Geometry: final body of the model. Coordinates: model frame, mm. Round coordinates to 2 decimals unless told otherwise and drop trailing zeros. Write each loop counter-clockwise with the first axis right and the second up, starting at its lowest first coordinate (ties: lowest second). Pieces come first, ordered by that corner, then holes. Notation, with made-up numbers: (65, -32) - (77, -32) arc R25 ccw to (77, 7) - close; hole circle Ø11 at (-23, -18.5). An arc over 180 degrees is marked (long way). Write each question's results on one line, items separated by ' | '.
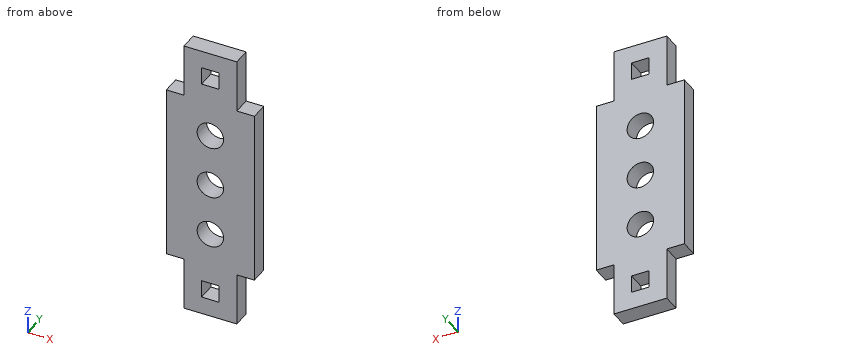
from build123d import *

# Parameters (mm, degrees)
CYLINDER005_R          = 2.25
CYLINDER005_DEPTH      = 3
CYLINDER005_ROLL_ANGLE = 90
CYLINDER006_R          = 2.25
CYLINDER006_DEPTH      = 3
CYLINDER006_ROLL_ANGLE = 90
CYLINDER004_R          = 2.25
CYLINDER004_DEPTH      = 3
CYLINDER004_ROLL_ANGLE = 90
BOX011_W               = 15
BOX011_H               = 3
BOX011_DEPTH           = 30
BOX010_W               = 3
BOX010_H               = 3
BOX010_DEPTH           = 3
BOX009_W               = 9
BOX009_H               = 3
BOX009_DEPTH           = 9
BOX013_W               = 3
BOX013_H               = 3
BOX013_DEPTH           = 3
BOX012_W               = 9
BOX012_H               = 3
BOX012_DEPTH           = 9


with BuildPart() as cylinder005:
    # Cylinder005 → Cylinder005 (new body)
    with BuildSketch(Plane.XY):
        Circle(CYLINDER005_R)
    extrude(amount=CYLINDER005_DEPTH)


with BuildPart() as cylinder005_1:
    # Cylinder005 roll: moved
    add(cylinder005.part.rotate(Axis((0, 0, 0), (1, 0, 0)), CYLINDER005_ROLL_ANGLE))


with BuildPart() as cylinder005_2:
    # Cylinder005 placement: moved
    add(cylinder005_1.part.moved(Location((0, -63, -3))))


with BuildPart() as cylinder006:
    # Cylinder006 → Cylinder006 (new body)
    with BuildSketch(Plane.XY):
        Circle(CYLINDER006_R)
    extrude(amount=CYLINDER006_DEPTH)


with BuildPart() as cylinder006_1:
    # Cylinder006 roll: moved
    add(cylinder006.part.rotate(Axis((0, 0, 0), (1, 0, 0)), CYLINDER006_ROLL_ANGLE))


with BuildPart() as cylinder006_2:
    # Cylinder006 placement: moved
    add(cylinder006_1.part.moved(Location((0, -63, -21))))


with BuildPart() as cylinder004:
    # Cylinder004 → Cylinder004 (new body)
    with BuildSketch(Plane.XY):
        Circle(CYLINDER004_R)
    extrude(amount=CYLINDER004_DEPTH)


with BuildPart() as cylinder004_1:
    # Cylinder004 roll: moved
    add(cylinder004.part.rotate(Axis((0, 0, 0), (1, 0, 0)), CYLINDER004_ROLL_ANGLE))


with BuildPart() as cylinder004_2:
    # Cylinder004 placement: moved
    add(cylinder004_1.part.moved(Location((0, -63, -12))))


with BuildPart() as cube011:
    # Box011 → Box011 (new body)
    with BuildSketch(Plane(origin=(-7.5, -66, -27), x_dir=(1, 0, 0), z_dir=(0, 0, 1))):
        with Locations((7.5, 1.5)):
            Rectangle(BOX011_W, BOX011_H)
    extrude(amount=BOX011_DEPTH)


with BuildPart() as cube010:
    # Box010 → Box010 (new body)
    with BuildSketch(Plane(origin=(-1.5, -66, 6), x_dir=(1, 0, 0), z_dir=(0, 0, 1))):
        with Locations((1.5, 1.5)):
            Rectangle(BOX010_W, BOX010_H)
    extrude(amount=BOX010_DEPTH)


with BuildPart() as cut010:
    # Box009 → Box009 (new body)
    with BuildSketch(Plane(origin=(-4.5, -66, 3), x_dir=(1, 0, 0), z_dir=(0, 0, 1))):
        with Locations((4.5, 1.5)):
            Rectangle(BOX009_W, BOX009_H)
    extrude(amount=BOX009_DEPTH)

    # Cut010: cut Cube010
    add(cube010.part, mode=Mode.SUBTRACT)


with BuildPart() as cube013:
    # Box013 → Box013 (new body)
    with BuildSketch(Plane(origin=(-1.5, -66, 6), x_dir=(1, 0, 0), z_dir=(0, 0, 1))):
        with Locations((1.5, 1.5)):
            Rectangle(BOX013_W, BOX013_H)
    extrude(amount=BOX013_DEPTH)


with BuildPart() as pitchringconnector:
    # Box012 → Box012 (new body)
    with BuildSketch(Plane(origin=(-4.5, -66, 3), x_dir=(1, 0, 0), z_dir=(0, 0, 1))):
        with Locations((4.5, 1.5)):
            Rectangle(BOX012_W, BOX012_H)
    extrude(amount=BOX012_DEPTH)

    # Cut011: cut Cube013
    add(cube013.part, mode=Mode.SUBTRACT)


with BuildPart() as pitchringconnector_1:
    # Cut011 placement: moved
    add(pitchringconnector.part.moved(Location((0, 0, -39))))

    # Fusion: union Cube011, Cut010
    add(cube011.part)
    add(cut010.part)

    # Cut012: cut Cylinder004
    add(cylinder004_2.part, mode=Mode.SUBTRACT)

    # Cut013: cut Cylinder006
    add(cylinder006_2.part, mode=Mode.SUBTRACT)

    # Cut014: cut Cylinder005
    add(cylinder005_2.part, mode=Mode.SUBTRACT)


with BuildPart() as pitchringconnector_2:
    # Cut014 placement: moved
    add(pitchringconnector_1.part.moved(Location((0, 29, -3))))


solid = pitchringconnector_2.part
Q1. Section query C-C, the plane y = -34.95. Return loops of the section in (x, z).
Answer block:
outline: (-7.5, -30) - (-4.5, -30) - (-4.5, -39) - (4.5, -39) - (4.5, -30) - (7.5, -30) - (7.5, 0) - (4.5, 0) - (4.5, 9) - (-4.5, 9) - (-4.5, 0) - (-7.5, 0) - close; hole circle Ø4.5 at (0, -24); hole circle Ø4.5 at (0, -15); hole circle Ø4.5 at (0, -6); hole (-1.5, -36) - (1.5, -36) - (1.5, -33) - (-1.5, -33) - close; hole (-1.5, 3) - (1.5, 3) - (1.5, 6) - (-1.5, 6) - close
Q2. Ray query, line 1 along Z through (x, y) = (0, -35.35); line 2 along Z through (x, y) = (-0.75, -35.2); line 3 along Z through (x, y) = (-7, -36.25). Return the intervals inside material, ascending.
Answer block:
line 1: -39 to -36, -33 to -26.25, -21.75 to -17.25, -12.75 to -8.25, -3.75 to 3, 6 to 9 | line 2: -39 to -36, -33 to -26.12, -21.88 to -17.12, -12.88 to -8.12, -3.88 to 3, 6 to 9 | line 3: -30 to 0
Q3. Section query D-D, the plane z = -15. Return loops of the section in (x, y).
Answer block:
outline: (-7.5, -37) - (-2.25, -37) - (-2.25, -34) - (-7.5, -34) - close; (2.25, -37) - (7.5, -37) - (7.5, -34) - (2.25, -34) - close
Q4. Section query B-B, the plane x = 0. Return loops of the section in (y, z).
Answer block:
outline: (-37, -39) - (-34, -39) - (-34, -36) - (-37, -36) - close; (-37, -33) - (-34, -33) - (-34, -26.25) - (-37, -26.25) - close; (-37, -21.75) - (-34, -21.75) - (-34, -17.25) - (-37, -17.25) - close; (-37, -12.75) - (-34, -12.75) - (-34, -8.25) - (-37, -8.25) - close; (-37, -3.75) - (-34, -3.75) - (-34, 3) - (-37, 3) - close; (-37, 6) - (-34, 6) - (-34, 9) - (-37, 9) - close
Q5. Pin query (flat end, axial travel): pin 1 (1.5 mm diameter, centred on y = -35, z = 6, fed in from -X); pin 2 (1.5 mm diameter, centred on x = 5.5, y = -35.5, fed in from -Z); pin 3 (6 mm diameter, centred on x = 0, z = -24, fed in from -Y); pin 4 (1.5 mm diameter, centred on y = -35.5, z = -35.5, fed in from +X). Return the tip coordinate at first contact, or that it passes through.
Answer block:
pin 1: x = -4.5 | pin 2: z = -30 | pin 3: y = -37 | pin 4: x = 4.5
Q6. Section query A-A, the plane z = -34. Return loops of the section in (x, y).
Answer block:
outline: (-4.5, -37) - (-1.5, -37) - (-1.5, -34) - (-4.5, -34) - close; (1.5, -37) - (4.5, -37) - (4.5, -34) - (1.5, -34) - close
